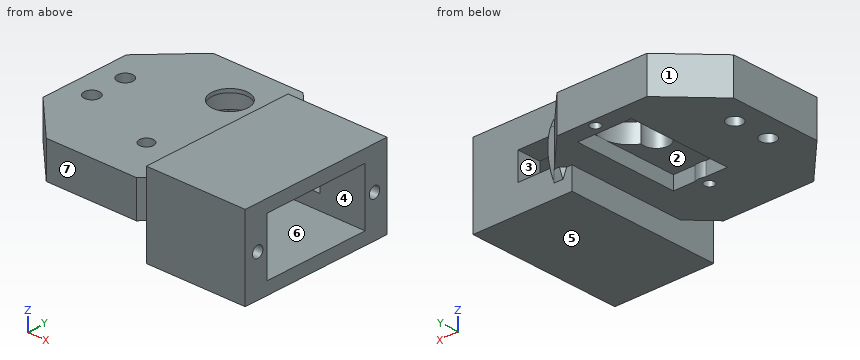
```python
from build123d import *

# Parameters (mm, degrees)
SKETCH_1_W                = 50
SKETCH_1_H                = 40
EXTRUDE_1_DEPTH           = 8
CHAMFER_1_SIZE            = 10
SKETCH_2_R                = 1.55
CUT_EXTRUDE_1_DEPTH       = 10
EXTRUDE_2_DEPTH           = 40
EXTRUDE_2_DEPTH_BACK      = 15
SKETCH_3_R                = 12.5
SKETCH_4_R                = 1.7
CUT_EXTRUDE_2_DEPTH       = 15
CUT_EXTRUDE_START         = -20
CUT_EXTRUDE_3_DEPTH       = 20
SKETCH_7_R                = 16.5
CUT_EXTRUDE_8_DEPTH       = 33
CUT_EXTRUDE_9_DEPTH       = 20
CHAMFER_3_SIZE            = 2
SKETCH_10_OUTSIDE_W       = 47.322
SKETCH_10_OUTSIDE_H       = 62.322
SKETCH_10_OUTSIDE_R       = 12.5
CUT_EXTRUDE_10_DEPTH      = 10
CHAMFER_4_SIZE            = 10
SKETCH_12_W               = 1.5
SKETCH_12_H               = 20
SKETCH_14_W               = 12
SKETCH_14_H               = 23
CUT_EXTRUDE_11_DEPTH      = 3
CUT_EXTRUDE_12_DEPTH      = 4.2
SKETCH_16_R               = 1.1
CUT_EXTRUDE_13_DEPTH      = 5
SKETCH_17_R               = 3.372674955
EXTRUDE_3_DEPTH           = 4
SKETCH_18_R               = 1.1
CUT_EXTRUDE_14_DEPTH      = 4
SKETCH_20_R               = 4
CUT_EXTRUDE_15_DEPTH      = 4
CUT_EXTRUDE_16_DEPTH      = 70.980354503
CUT_EXTRUDE_16_DEPTH_BACK = 70.980354503
SKETCH_21_W               = 56.3061188
SKETCH_21_H               = 46.683670243
EXTRUDE_4_DEPTH           = 18
EXTRUDE_4_DEPTH_BACK      = 4
SKETCH_22_W               = 18
SKETCH_22_H               = 34
SKETCH_23_W               = 12.5
SKETCH_23_H               = 23.5
CUT_EXTRUDE_17_DEPTH      = 18
SKETCH_24_R               = 1.25
CUT_EXTRUDE_18_DEPTH      = 8
CUT_EXTRUDE_19_DEPTH      = 64.641574462
SKETCH_26_W               = 8
SKETCH_26_H               = 6
CUT_EXTRUDE_20_DEPTH      = 20


# Read off the part's stored shape, not the designer's step: 切除-拉伸3
with BuildPart() as part:
    # 草图1 → 凸台-拉伸1 (new body)
    with BuildSketch(Plane.XY):
        Rectangle(SKETCH_1_W, SKETCH_1_H)
    extrude(amount=EXTRUDE_1_DEPTH)

    # 倒角1
    chamfer_1_edges = [part.edges().sort_by_distance(p)[0] for p in [
        (-25, -20, 4),
        (-25, 20, 4),
    ]]
    chamfer(chamfer_1_edges, length=CHAMFER_1_SIZE)

    # 草图2 → 切除-拉伸1 (cut)
    with BuildSketch(Plane.XY.offset(8)):
        with Locations((-2, -10)):
            Circle(SKETCH_2_R)
        with Locations((-2, 10)):
            Circle(SKETCH_2_R)
    extrude(amount=-CUT_EXTRUDE_1_DEPTH, mode=Mode.SUBTRACT)

    # 草图3 → 凸台-拉伸2 (add, two sides: drawn at the far end of the back side and taken through both)
    with BuildSketch(Plane(origin=(25, 0, 0), x_dir=(0, 0, -1), z_dir=(1, 0, 0)).offset(-EXTRUDE_2_DEPTH_BACK)):
        with Locations(Location((-4, 0, 0), (0, 0, 251.337075115))):
            Circle(SKETCH_3_R)
    extrude(amount=EXTRUDE_2_DEPTH + EXTRUDE_2_DEPTH_BACK)

    # 草图4 → 切除-拉伸2 (cut)
    with BuildSketch(Plane.XY.offset(8)):
        with Locations((-19.690178066, -4)):
            Circle(SKETCH_4_R)
        with Locations((-19.690178066, 4)):
            Circle(SKETCH_4_R)
    extrude(amount=-CUT_EXTRUDE_2_DEPTH, mode=Mode.SUBTRACT)

    # 切除-拉伸3 outline → 切除-拉伸3 (cut)
    with BuildSketch(Plane(origin=(65, 0, 0), x_dir=(0, 0, -1), z_dir=(1, 0, 0)).offset(CUT_EXTRUDE_START)):
        with BuildLine():
            Line((7.456439237, -5), (-15.456439237, -5))
            ThreePointArc((-15.456439237, -5), (-4, -12.5), (7.456439237, -5))
        make_face()
        with BuildLine():
            ThreePointArc((7.456439237, 5), (-4, 12.5), (-15.456439237, 5))
            Line((-15.456439237, 5), (7.456439237, 5))
        make_face()
    extrude(amount=CUT_EXTRUDE_3_DEPTH, mode=Mode.SUBTRACT)

    # 草图7 → 切除-拉伸8 (cut)
    with BuildSketch(Plane.XZ.offset(5)):
        with Locations((48.5, 4)):
            Circle(SKETCH_7_R)
    cut_extrude_8 = extrude(amount=CUT_EXTRUDE_8_DEPTH, mode=Mode.SUBTRACT)

    # 镜向1: 切除-拉伸8 across plane
    add(cut_extrude_8.mirror(Plane.ZX), mode=Mode.SUBTRACT)

    # 草图8 → 切除-拉伸9 (cut)
    with BuildSketch(Plane.XZ.offset(5)):
        with BuildLine():
            Line((50, 19.107397707), (75.764252489, 33.62580965))
            Line((75.764252489, 33.62580965), (78.826270749, -18.347337912))
            Line((78.826270749, -18.347337912), (50, -10.892602293))
            ThreePointArc((50, -10.892602293), (65, 4.107397707), (50, 19.107397707))
        make_face()
    extrude(amount=-CUT_EXTRUDE_9_DEPTH, mode=Mode.SUBTRACT)

    # 倒角3
    chamfer_3_edges = [part.edges().sort_by_distance(p)[0] for p in [
        (10, 0, 16.5),
        (10, 0, -8.5),
    ]]
    chamfer(chamfer_3_edges, length=CHAMFER_3_SIZE)

    # 草图10 outside → 切除-拉伸10 (cut)
    with BuildSketch(Plane(origin=(25, 0, 0), x_dir=(0, 0, -1), z_dir=(1, 0, 0))):
        with Locations((-4, 0)):
            Rectangle(SKETCH_10_OUTSIDE_W, SKETCH_10_OUTSIDE_H)
        with Locations((-4.107397707, 0)):
            Circle(SKETCH_10_OUTSIDE_R, mode=Mode.SUBTRACT)
    extrude(amount=-CUT_EXTRUDE_10_DEPTH, mode=Mode.SUBTRACT)

    # 倒角4
    # the kernel refuses this chamfer: 10 mm, written as the material it takes off along each edge
    with BuildSketch(Plane(origin=(15, -20, -25.71682988), x_dir=(-0.9996219169112968, -0.027495876610586317, 0), z_dir=(0, 0, 1))) as chamfer_4_piece_1_section:
        Polygon((CHAMFER_4_SIZE * 0.999621916911, -CHAMFER_4_SIZE * 0.0274958766106), (-CHAMFER_4_SIZE * 0.0274958766106, -CHAMFER_4_SIZE * 0.999621916911), (0, 0), align=None)
    chamfer_4_piece_1 = extrude(amount=59.433659759, mode=Mode.PRIVATE)
    chamfer_4_piece_1 = chamfer_4_piece_1 - Plane(origin=(11.669205873, 0, 4.107397707), x_dir=(0, 0, -1), z_dir=(1, 0, 0)) * Cylinder(12.5, 159, mode=Mode.PRIVATE)
    add(chamfer_4_piece_1, mode=Mode.SUBTRACT)
    with BuildSketch(Plane(origin=(15, 20, 33.71682988), x_dir=(-0.9996219169112968, 0.027495876610586317, 0), z_dir=(0, 0, -1))) as chamfer_4_piece_2_section:
        Polygon((CHAMFER_4_SIZE * 0.999621916911, -CHAMFER_4_SIZE * 0.0274958766106), (-CHAMFER_4_SIZE * 0.0274958766106, -CHAMFER_4_SIZE * 0.999621916911), (0, 0), align=None)
    chamfer_4_piece_2 = extrude(amount=59.433659759, mode=Mode.PRIVATE)
    chamfer_4_piece_2 = chamfer_4_piece_2 - Plane(origin=(11.669205873, 0, 4.107397707), x_dir=(0, 0, -1), z_dir=(1, 0, 0)) * Cylinder(12.5, 159, mode=Mode.PRIVATE)
    add(chamfer_4_piece_2, mode=Mode.SUBTRACT)

    # 草图12 → 切除-旋转2 (revolve, cut)
    with BuildSketch(Plane(origin=(0, 0, 0), x_dir=(1, 0, 0), z_dir=(0, 1, 0))):
        with Locations((14.75, 8.392602293)):
            Rectangle(SKETCH_12_W, SKETCH_12_H)
    revolve(axis=Axis((50, 0, 4.107397707), (-1, 0, 0)), mode=Mode.SUBTRACT)

    # 草图14 → 切除-拉伸11 (cut)
    with BuildSketch(Plane(origin=(0, 0, 0), x_dir=(-1, 0, 0), z_dir=(0, 0, -1))):
        with Locations((2, 4.65)):
            Rectangle(SKETCH_14_W, SKETCH_14_H)
    extrude(amount=-CUT_EXTRUDE_11_DEPTH, mode=Mode.SUBTRACT)

    # 草图15 → 切除-拉伸12 (cut)
    with BuildSketch(Plane(origin=(0, 0, 3), x_dir=(-1, 0, 0), z_dir=(0, 0, -1))):
        with BuildLine():
            ThreePointArc((4.631967524, 4.49702381), (2, 16.1), (-0.631967524, 4.49702381))
            ThreePointArc((-0.631967524, 4.49702381), (2, 0.95), (4.631967524, 4.49702381))
        make_face()
    extrude(amount=-CUT_EXTRUDE_12_DEPTH, mode=Mode.SUBTRACT)

    # 草图16 → 切除-拉伸13 (cut)
    with BuildSketch(Plane(origin=(0, 0, 0), x_dir=(-1, 0, 0), z_dir=(0, 0, -1))):
        with Locations((2, 18.3)):
            Circle(SKETCH_16_R)
    extrude(amount=-CUT_EXTRUDE_13_DEPTH, mode=Mode.SUBTRACT)

    # 草图17 → 凸台-拉伸3 (add)
    with BuildSketch(Plane(origin=(0, 0, 0), x_dir=(-1, 0, 0), z_dir=(0, 0, -1))):
        with Locations((2, -10)):
            Circle(SKETCH_17_R)
    extrude(amount=-EXTRUDE_3_DEPTH)

    # 草图18 → 切除-拉伸14 (cut)
    with BuildSketch(Plane(origin=(0, 0, 0), x_dir=(-1, 0, 0), z_dir=(0, 0, -1))):
        with Locations((2, -9)):
            Circle(SKETCH_18_R)
    extrude(amount=-CUT_EXTRUDE_14_DEPTH, mode=Mode.SUBTRACT)

    # 草图20 → 切除-拉伸15 (cut)
    with BuildSketch(Plane(origin=(0, 0, 7.2), x_dir=(-1, 0, 0), z_dir=(0, 0, -1))):
        with Locations((2, 10)):
            Circle(SKETCH_20_R)
    extrude(amount=-CUT_EXTRUDE_15_DEPTH, mode=Mode.SUBTRACT)

    # 草图21 → 切除-拉伸16 (cut, two sides: drawn at the far end of the back side and taken through both)
    with BuildSketch(Plane(origin=(0, 0, 0), x_dir=(-1, 0, 0), z_dir=(0, 0, -1)).offset(-CUT_EXTRUDE_16_DEPTH_BACK)):
        with Locations((-42.1530594, 7.959183123)):
            Rectangle(SKETCH_21_W, SKETCH_21_H)
    extrude(amount=CUT_EXTRUDE_16_DEPTH + CUT_EXTRUDE_16_DEPTH_BACK, mode=Mode.SUBTRACT)

    # 草图22 → 凸台-拉伸4 (add, two sides: drawn at the far end of the back side and taken through both)
    with BuildSketch(Plane(origin=(14, 0, 0), x_dir=(0, 0, -1), z_dir=(1, 0, 0)).offset(-EXTRUDE_4_DEPTH_BACK)):
        with Locations((-4.107397707, -6)):
            Rectangle(SKETCH_22_W, SKETCH_22_H)
    extrude(amount=EXTRUDE_4_DEPTH + EXTRUDE_4_DEPTH_BACK)

    # 草图23 → 切除-拉伸17 (cut)
    with BuildSketch(Plane(origin=(32, 0, 0), x_dir=(0, 0, -1), z_dir=(1, 0, 0))):
        with Locations((-4.107397707, -6)):
            Rectangle(SKETCH_23_W, SKETCH_23_H)
    extrude(amount=-CUT_EXTRUDE_17_DEPTH, mode=Mode.SUBTRACT)

    # 草图24 → 切除-拉伸18 (cut)
    with BuildSketch(Plane(origin=(32, 0, 0), x_dir=(0, 0, -1), z_dir=(1, 0, 0))):
        with Locations((-4.107397707, 8)):
            Circle(SKETCH_24_R)
        with Locations(Location((-4.107397707, -20, 0), (0, 0, 180))):
            Circle(SKETCH_24_R)
    extrude(amount=-CUT_EXTRUDE_18_DEPTH, mode=Mode.SUBTRACT)

    # 草图25 → 切除-拉伸19 (cut, through all)
    with BuildSketch(Plane(origin=(32, 0, 0), x_dir=(0, 0, -1), z_dir=(1, 0, 0))):
        with BuildLine():
            Line((-13.107397707, -8.561851845), (-13.107397707, 8.561851845))
            ThreePointArc((-13.107397707, 8.561851845), (-16.5, 0), (-13.107397707, -8.561851845))
        make_face()
        with BuildLine():
            Line((4.892602293, -8.784738155), (4.892602293, 8.784738155))
            ThreePointArc((4.892602293, 8.784738155), (8.5, 0), (4.892602293, -8.784738155))
        make_face()
    extrude(amount=-CUT_EXTRUDE_19_DEPTH, mode=Mode.SUBTRACT)

    # 草图26 → 切除-拉伸20 (cut)
    with BuildSketch(Plane.XZ.offset(-5.75)):
        with Locations((18, 4.107397707)):
            Rectangle(SKETCH_26_W, SKETCH_26_H)
    extrude(amount=-CUT_EXTRUDE_20_DEPTH, mode=Mode.SUBTRACT)


solid = part.part
```
Here's how the part is built. I have some questions about the finished solid (model axes, mm). Face numbers are marked on the shaded views. A direction names the side the tool comes from. Give positions to 0.01 mm unless a question says otherwise; leave off trailing zeros. Order: outer loops, then holes, each group sorted by start corner. A loop starts at its lowest first (then second) coordinate and runs counter-clockwise, first axis right, second up. Notation, with made-up numbers: (67.25, 67.25) -> (89.25, 67.25) arc R9 ccw to (89.25, 73.25) -> close; hole circle Ø1 at (34.5, 20). An arc over 180 degrees is marked (long way). Use CSV: the item, a comma, the result in double quotes. Start each with the question number.
Item 1: Suppose I cut it at A-A (x = 29). List the corners of the cut face in (y, z) for me, and give its area (3 significant figures).
Item 2: Thinking about a two-plate mould opening in Z: for the marked faces 5, 6 and 7, which applies, pulls with the +Z half, pulls with the -Z half, needs draft (parallel to the pull), parting line crosses it, or undercut?
Item 3: Suppose I cut it at C-C (x = 15). List the corners of the cut face in (y, z) for me.
Item 4: Suppose I cut it at B-B (y = -4). List the corners of the cut face in (x, z) for me.
Item 5: If I drill on probe 1 along Y at (x, z) = (-2, 3.5); probe 2 along Y at (x, z) = (-2, 5.75); probe 3 along Z at (x, y) = (29, -5), over which ranges is the centre line in solid material (lowest first)? Write a range as [from, to].
Item 6: On a 3-axis mill with a long thin cutter (end or side, diameter ignored), from which of +Z, -Z, +X, -X, +Y, -Y can I reach the whole of each face in a straight line? I mean the marked faces 1, 2, 3 and 4. Say none if no direction works.
Item 7: Suppose I cut it at D-D (x = 6.5). List the corners of the cut face in (y, z) for me.
Item 8: I'm going to push flat-ended pins straight in: P1, Ø1.5, axis at y = 3.5, z = 2, coming from the +X side; P2, Ø1.5, axis at x = -2, z = 0, coming from the -Y side; P3, Ø10, axis at x = 26, z = 2, coming from the +Y side. Where does each tip first touch, or does it pass through?
Answer block:
1,outline,"(-23, -4.89) -> (11, -4.89) -> (11, 13.11) -> (-23, 13.11) -> close; hole circle Ø2.5 at (-20, 4.11); hole (-17.75, -2.14) -> (5.75, -2.14) -> (5.75, 10.36) -> (-17.75, 10.36) -> close; hole circle Ø2.5 at (8, 4.11)"
1,area,"308 mm^2"
2,face 5,"pulls with the -Z half"
2,face 6,"undercut"
2,face 7,"needs draft"
3,outline,"(-23, -4.89) -> (11, -4.89) -> (11, 1.11) -> (5.75, 1.11) -> (5.75, -2.14) -> (-17.75, -2.14) -> (-17.75, 10.36) -> (5.75, 10.36) -> (5.75, 7.11) -> (11, 7.11) -> (11, 13.11) -> (-23, 13.11) -> close"
4,outline,"(-25, 0) -> (-21.39, 0) -> (-21.39, 8) -> (-25, 8) -> close; (-17.99, 0) -> (-8, 0) -> (-8, 3) -> (4, 3) -> (4, 0) -> (10, 0) -> (10, -4.89) -> (32, -4.89) -> (32, -2.14) -> (14, -2.14) -> (14, 10.36) -> (32, 10.36) -> (32, 13.11) -> (10, 13.11) -> (10, 8) -> (-17.99, 8) -> close"
5,probe 1,"y = [-20, -10.1], [-7.9, 0.95], [16.1, 17.2], [19.4, 20]"
5,probe 2,"y = [-20, -11.55], [-8.45, 0.95], [16.1, 20]"
5,probe 3,"z = [-4.89, -2.14], [10.36, 13.11]"
6,face 1,"+Z, -Z, -X, +Y"
6,face 2,"-Z"
6,face 3,"+Y"
6,face 4,"+X"
7,outline,"(-18.5, 0) -> (18.5, 0) -> (18.5, 8) -> (-18.5, 8) -> close"
8,P1,"stops at x = 14"
8,P2,"stops at y = -20"
8,P3,"stops at y = 11"
